from build123d import *

# Parameters (mm, degrees)
SKETCH_1_R          = 26
SKETCH_1_R_2        = 20
EXTRUDE_1_DEPTH     = 3.5
SKETCH_2_R          = 23.523275985
SKETCH_2_R_2        = 22.187065931
CUT_EXTRUDE_3_DEPTH = 2


with BuildPart() as part:
    # 草图1 → 凸台-拉伸1 (new, symmetric)
    with BuildSketch(Plane.XY):
        Circle(SKETCH_1_R)
        Circle(SKETCH_1_R_2, mode=Mode.SUBTRACT)
    extrude(amount=EXTRUDE_1_DEPTH, both=True)

    # 草图2 → 切除-拉伸3 (cut)
    with BuildSketch(Plane.XY.offset(3.5)):
        Circle(SKETCH_2_R)
        Circle(SKETCH_2_R_2, mode=Mode.SUBTRACT)
    extrude(amount=-CUT_EXTRUDE_3_DEPTH, mode=Mode.SUBTRACT)


solid = part.part
Geometry check sheet. Reference: the model listing, model coordinates, mm. A direction names the side the tool comes from. Round coordinates to 2 decimals unless told otherwise and drop trailing zeros. Order: outer loops, then holes, each group sorted by start corner. A loop starts at its lowest first (then second) coordinate and runs counter-clockwise, first axis right, second up. Notation, with made-up numbers: M -30,82.5 L 21,82.5 A34 ccw 21,118.5 Z; hole C -28.75,19 d6. An arc over 180 degrees is marked long. Answer in a Markdown table with one row per item. Add a question column.
Item 1: Draft check along Y on faces 3 (the face through (-6, -23, 3.5)), 4 (the face through (-20.633, -15.821, 0.049)), 5 (the face through (22.437, 7.066, 2.514)). Enter one of: released by +Y, released by -Y, zero draft, split by the parting line, or undercut.
Item 2: Set-up check for faces 1 (the face through (21.163, 6.664, 2.514)), 2 (the face through (-4.336, -19.524, -0.049)): record each of +Z, -Z, +X, -X, +Y, -Y from which the full face is reachable in a straight line by a thin tool's end or side.
Item 3: Depth check by flat-ended pin: pin 1 Ø1.5 at (x, z) = (-17, 0.5) entering from +Y; pin 2 Ø2 at (x, y) = (19.5, 20.5) entering from +Z; pin 3 Ø3 at (y, z) = (2, -1.5) entering from -X; pin 4 Ø2 at (y, z) = (-4.5, -2.5) entering from -X. Enter the tip coordinate at first touch or a pass-through.
Item 4: Sectioned sample at D-D, the plane y = -21.5. Enter the section's corners in (x, z).
Item 5: Sectioned sample at C-C, the plane z = 0. Enter the section's corners in (x, y), plus the area to 3 significant figures.
Item 6: Material ranges on L1, parallel to Y at x = 0, z = 2.1; L2, parallel to Y at x = 0, z = -0.5; L3, parallel to X at y = 11, z = 2.25, recorded low to high. Write a range as [from, to].
Item 7: Sectioned sample at A-A, the plane x = 0. Enter the section's corners in (y, z).
Filled in:
| question | item | result |
|---|---|---|
| 1 | face 3 | zero draft |
| 1 | face 4 | split by the parting line |
| 1 | face 5 | undercut |
| 2 | face 1 | +Z |
| 2 | face 2 | +Z, -Z |
| 3 | pin 1 | stops at y = 20.3 |
| 3 | pin 2 | passes through |
| 3 | pin 3 | stops at x = -26 |
| 3 | pin 4 | stops at x = -25.76 |
| 4 | outline | M -14.62,-3.5 L 14.62,-3.5 L 14.62,3.5 L 9.54,3.5 L 9.54,1.5 L 5.48,1.5 L 5.48,3.5 L -5.48,3.5 L -5.48,1.5 L -9.54,1.5 L -9.54,3.5 L -14.62,3.5 Z |
| 5 | outline | C 0,0 d52; hole C 0,0 d40 |
| 5 | area | 867 mm² |
| 6 | L1 | y = [-26, -23.52], [-22.19, -20], [20, 22.19], [23.52, 26] |
| 6 | L2 | y = [-26, -20], [20, 26] |
| 6 | L3 | x = [-23.56, -20.79], [-19.27, -16.7], [16.7, 19.27], [20.79, 23.56] |
| 7 | outline | M -26,-3.5 L -20,-3.5 L -20,3.5 L -22.19,3.5 L -22.19,1.5 L -23.52,1.5 L -23.52,3.5 L -26,3.5 Z; M 20,-3.5 L 26,-3.5 L 26,3.5 L 23.52,3.5 L 23.52,1.5 L 22.19,1.5 L 22.19,3.5 L 20,3.5 Z |
